Source: CAD feature listing. Evaluate the final solid. Frame: model axes, mm. A direction names the side the tool comes from. Give positions to 0.01 mm unless a question says otherwise; leave off trailing zeros. Order: outer loops, then holes, each group sorted by start corner. A loop starts at its lowest first (then second) coordinate and runs counter-clockwise, first axis right, second up. Notation, with made-up numbers: (71, 50) - (104, 50) arc R21 ccw to (104, 64) - close; hole circle Ø7 at (-1, 50.25). An arc over 180 degrees is marked (long way). Use CSV: the item, a comma, the result in double quotes.
```python
from build123d import *

# Parameters (mm, degrees)
BOSS_EXTRUDE1_DEPTH = 79
SKETCH2_R           = 5
CUT_EXTRUDE1_DEPTH  = 95.292099351
CUT_EXTRUDE3_DEPTH  = 95.292099351
FILLET1_R           = 1.5
SKETCH5_R           = 1.25
CUT_EXTRUDE4_DEPTH  = 95.292099351


with BuildPart() as part:
    # Sketch1 → Boss-Extrude1 (new body)
    with BuildSketch(Plane(origin=(0, 0, 0), x_dir=(1, 0, 0), z_dir=(0, 1, 0))):
        Polygon((0, 0), (0, -2), (23, -2), (23, -45), (25, -45), (25, 0), align=None)
    extrude(amount=BOSS_EXTRUDE1_DEPTH)

    # Sketch2 → Cut-Extrude1 (cut, through all)
    with BuildSketch(Plane(origin=(25, 0, 0), x_dir=(0, 0, -1), z_dir=(1, 0, 0))):
        with Locations((-31, 39.5)):
            Circle(SKETCH2_R)
    extrude(amount=-CUT_EXTRUDE1_DEPTH, mode=Mode.SUBTRACT)

    # Sketch3 → Cut-Extrude3 (cut, through all)
    with BuildSketch(Plane(origin=(25, 0, 0), x_dir=(0, 0, -1), z_dir=(1, 0, 0))):
        Polygon((-56.02971798, 54), (-45, 54), (-45, 79), (-20, 79), (-20, 83.569029918), (-56.02971798, 83.569029918), align=None)
        Polygon((-45, 0), (-45, 25), (-50.640365422, 25), (-50.640365422, -10.402653787), (-20, -10.402653787), (-20, 0), align=None)
        with BuildLine():
            ThreePointArc((-20, 0), (-37.67766953, 7.32233047), (-45, 25))
            Line((-45, 25), (-45, 0))
            Line((-45, 0), (-20, 0))
        make_face()
        with BuildLine():
            Line((-45, 79), (-45, 54))
            ThreePointArc((-45, 54), (-37.67766953, 71.67766953), (-20, 79))
            Line((-20, 79), (-45, 79))
        make_face()
    extrude(amount=-CUT_EXTRUDE3_DEPTH, mode=Mode.SUBTRACT)

    # Fillet1
    fillet1_edges = [part.edges().sort_by_distance(p)[0] for p in [
        (25, 39.5, 0),
        (23, 39.5, 2),
    ]]
    fillet(fillet1_edges, radius=FILLET1_R)

    # Sketch5 → Cut-Extrude4 (cut, through all)
    with BuildSketch(Plane(origin=(0, 0, 0), x_dir=(-1, 0, 0), z_dir=(0, 0, -1))):
        with Locations((-18, 69.5)):
            Circle(SKETCH5_R)
        with Locations((-9, 69.5)):
            Circle(SKETCH5_R)
        with Locations((-9, 9.5)):
            Circle(SKETCH5_R)
        with Locations((-18, 9.5)):
            Circle(SKETCH5_R)
    extrude(amount=-CUT_EXTRUDE4_DEPTH, mode=Mode.SUBTRACT)


solid = part.part
```
Item 1: Section B-B on y = 69.5. Return the cut outline in (x, z), then the cut area to 3 significant figures.
Filled in:
outline,"(0, 0) - (7.75, 0) - (7.75, 2) - (0, 2) - close; (10.25, 0) - (16.75, 0) - (16.75, 2) - (10.25, 2) - close; (19.25, 0) - (23.5, 0) arc R1.5 ccw to (25, 1.5) - (25, 39.62) - (23, 39.62) - (23, 3.5) arc R1.5 cw to (21.5, 2) - (19.25, 2) - close"
area,"115 mm2"
Item 2: Section C-C on x = 2. Return the cut outline in (y, z).
Filled in:
outline,"(0, 0) - (79, 0) - (79, 2) - (0, 2) - close"
Item 3: First-contact query: pin 1 (13 mm diameter, centred on y = 39.5, z = 31, fed in from +X); pin 2 (3 mm diameter, centred on x = 22, z = 28, fed in from +Y); pin 3 (6.5 mm diameter, centred on x = 10.5, y = 25.5, fed in from +Z). Flat tips, straight axial feed; report the tip coordinate or a pass-through.
Filled in:
pin 1,"stops at x = 25"
pin 2,"stops at y = 78.03"
pin 3,"stops at z = 2"
Item 4: Section A-A on x = 9. Return the cut outline in (y, z), then the cut area to 3 significant figures.
Filled in:
outline,"(0, 0) - (8.25, 0) - (8.25, 2) - (0, 2) - close; (10.75, 0) - (68.25, 0) - (68.25, 2) - (10.75, 2) - close; (70.75, 0) - (79, 0) - (79, 2) - (70.75, 2) - close"
area,"148 mm2"
Item 5: Material intervals for line 1 (Y direction, x = 9, z = 0.65); line 2 (Z direction, x = 9, y = 68); line 3 (X direction, y = 25, z = 21.5), sorted ascending. Write a range as from..to.
Filled in:
line 1,"y = 0..8.25, 10.75..68.25, 70.75..79"
line 2,"z = 0..2"
line 3,"x = 23..25"
Item 6: Set-up query: faces 5 (the flat face through (0, 39, 1)), 6 (the flat face through (11, 39, 2)). Return all of +Z, -Z, +X, -X, +Y, -Y with unobstructed straight access to the full face (end or side cutting, diameter ignored); none if empty.
Filled in:
face 5,"+Z, -Z, -X, +Y, -Y"
face 6,"+Z, -X, +Y, -Y"
Item 7: Mould query, pull axis Y, two halves, no side actions, for faces 1 (the cylindrical face through (17.328, 70.554, 0.986)), 2 (the flat face through (12, 39, 0)), 3 (the cylindrical face through (9.921, 10.345, 0.986)), 4 (the cylindrical face through (24.014, 71.482, 37.871)). Classes: released by +Y, released by -Y, zero draft, split by the parting line, or undercut.
Filled in:
face 1,"undercut"
face 2,"zero draft"
face 3,"undercut"
face 4,"released by +Y"
Item 8: Section D-D on z = 16. Return the cut outline in (x, y), then the cut area to 3 significant figures.
Filled in:
outline,"(23, 0) - (25, 0) - (25, 79) - (23, 79) - close"
area,"158 mm2"
